```python
from build123d import *

# Parameters (mm, degrees)
SKETCH1_W           = 127
SKETCH1_H           = 87
BOSS_EXTRUDE1_DEPTH = 1.5
SKETCH3_W           = 131
SKETCH3_H           = 91
SKETCH3_W_2         = 127
SKETCH3_H_2         = 87
BOSS_EXTRUDE2_DEPTH = 20
CUT_EXTRUDE1_REACH  = 115.891
SKETCH4_W           = 25
SKETCH4_H           = 10
CUT_EXTRUDE2_REACH  = 142.112
SKETCH5_W           = 11
SKETCH5_H           = 10
CUT_EXTRUDE3_DEPTH  = 1.5


with BuildPart() as part:
    # Sketch1 → Boss-Extrude1 (new body)
    with BuildSketch(Plane(origin=(0, 0, 0), x_dir=(1, 0, 0), z_dir=(0, 1, 0))):
        Rectangle(SKETCH1_W, SKETCH1_H)
    extrude(amount=BOSS_EXTRUDE1_DEPTH)

    # Sketch3 → Boss-Extrude2 (add)
    with BuildSketch(Plane(origin=(0, 0, 0), x_dir=(1, 0, 0), z_dir=(0, 1, 0))):
        Rectangle(SKETCH3_W, SKETCH3_H)
        Rectangle(SKETCH3_W_2, SKETCH3_H_2, mode=Mode.SUBTRACT)
    extrude(amount=BOSS_EXTRUDE2_DEPTH)

    # Sketch4 → Cut-Extrude1 (cut, up to next)
    with BuildSketch(Plane.XY.offset(45.5), mode=Mode.PRIVATE) as cut_extrude1_sk1:
        with Locations((-45, 17)):
            Rectangle(SKETCH4_W, SKETCH4_H)
    cut_extrude1_tool1 = extrude(cut_extrude1_sk1.sketch, amount=-CUT_EXTRUDE1_REACH, mode=Mode.PRIVATE) & part.part
    add(cut_extrude1_tool1.solids().sort_by_distance((-45, 17, 45.5))[0], mode=Mode.SUBTRACT)

    # Sketch5 → Cut-Extrude2 (cut, up to next)
    with BuildSketch(Plane(origin=(65.5, 0, 0), x_dir=(0, 0, -1), z_dir=(1, 0, 0)), mode=Mode.PRIVATE) as cut_extrude2_sk1:
        with Locations((27.5, 11)):
            Rectangle(SKETCH5_W, SKETCH5_H)
    cut_extrude2_tool1 = extrude(cut_extrude2_sk1.sketch, amount=-CUT_EXTRUDE2_REACH, mode=Mode.PRIVATE) & part.part
    add(cut_extrude2_tool1.solids().sort_by_distance((65.5, 11, -27.5))[0], mode=Mode.SUBTRACT)

    # Sketch6 → Cut-Extrude3 (cut)
    with BuildSketch(Plane(origin=(0, 20, 0), x_dir=(1, 0, 0), z_dir=(0, 1, 0))):
        Polygon((-57.5, -44.5), (-64.5, -44.5), (-64.5, 44.5), (64.5, 44.5), (64.5, -44.5), (-32.5, -44.5), (-32.5, -45.5), (65.5, -45.5), (65.5, 45.5), (-65.5, 45.5), (-65.5, -45.5), (-57.5, -45.5), align=None)
    extrude(amount=-CUT_EXTRUDE3_DEPTH, mode=Mode.SUBTRACT)


solid = part.part
```
The listing builds one solid part. Answer for the finished solid, in the listing's coordinates (mm). A direction names the side the tool comes from. Coordinates: 2 decimals unless noted, no trailing zeros. Loops run counter-clockwise (first coordinate to the right, second up) from the corner with the lowest first, then second, coordinate; pieces in that order, holes last. Notation, with made-up numbers: (24, -35.75) - (30, -35.75) arc R4 cw to (30, -31.75) - close; hole circle Ø5 at (74.25, 76.25). An arc over 180 degrees is marked (long way). Use a Markdown table: item, result. Add a question column.
1) The part is cut by section C-C, the plane x = 49. Give the vertices of the cut face in (y, z).
2) The part is cut by section B-B, the plane z = -30.5. Give the vertices of the cut face in (x, y), and give its area (4 significant figures).
3) The part is cut by section D-D, the plane z = 4. Give the vertices of the cut face in (x, y).
4) The mould has two halves that part along Z. Classify faces 3 (the flat face through (-1, 9, 45.5)), 4 (the flat face through (-1, 0, -1)), 5 (the flat face through (63.5, 11, 1)): released by +Z, released by -Z, zero draft, split by the parting line, or undercut.
5) The part is cut by section A-A, the plane y = 13.75. Give the vertices of the cut face in (x, z), and give its area (3 significant figures).
6) Find the intervals of material crossed by line 1 (Z direction, x = 45, y = 17.25); line 2 (X direction, y = 9.25, z = 31); line 3 (Z direction, x = 35, y = 19), in increasing order.
7) Given pin 1 (2 mm diameter, centred on x = 28, z = -25, fed in from +Y); pin 2 (1.6 mm diameter, centred on y = 19.5, z = 8.5, fed in from +X); pin 3 (1.6 mm diameter, centred on x = -62, y = 19.5, fed in from +Z), each flat-ended and moving along its own axis, determine where each tip first touches the part or whether it passes through.
8) For faces 1 (the flat face through (-1, 11, 43.5)), 2 (the flat face through (-1, 9, -45.5)), determine the directions among +Z, -Z, +X, -X, +Y, -Y from which every point of the face is accessible in a straight line to the end or side of a thin tool.
Here are the results:
| question | item | result |
|---|---|---|
| 1 | outline | (0, -45.5) - (18.5, -45.5) - (18.5, -44.5) - (20, -44.5) - (20, -43.5) - (1.5, -43.5) - (1.5, 43.5) - (20, 43.5) - (20, 44.5) - (18.5, 44.5) - (18.5, 45.5) - (0, 45.5) - close |
| 2 | outline | (-65.5, 0) - (65.5, 0) - (65.5, 6) - (63.5, 6) - (63.5, 1.5) - (-63.5, 1.5) - (-63.5, 20) - (-64.5, 20) - (-64.5, 18.5) - (-65.5, 18.5) - close; (63.5, 16) - (65.5, 16) - (65.5, 18.5) - (64.5, 18.5) - (64.5, 20) - (63.5, 20) - close |
| 2 | area | 247.5 mm^2 |
| 3 | outline | (-65.5, 0) - (65.5, 0) - (65.5, 18.5) - (64.5, 18.5) - (64.5, 20) - (63.5, 20) - (63.5, 1.5) - (-63.5, 1.5) - (-63.5, 20) - (-64.5, 20) - (-64.5, 18.5) - (-65.5, 18.5) - close |
| 4 | face 3 | released by +Z |
| 4 | face 4 | zero draft |
| 4 | face 5 | undercut |
| 5 | outline | (-65.5, -45.5) - (65.5, -45.5) - (65.5, -33) - (63.5, -33) - (63.5, -43.5) - (-63.5, -43.5) - (-63.5, 43.5) - (-57.5, 43.5) - (-57.5, 45.5) - (-65.5, 45.5) - close; (-32.5, 43.5) - (63.5, 43.5) - (63.5, -22) - (65.5, -22) - (65.5, 45.5) - (-32.5, 45.5) - close |
| 5 | area | 800 mm^2 |
| 6 | line 1 | z = -45.5 to -43.5, 43.5 to 45.5 |
| 6 | line 2 | x = -65.5 to -63.5, 63.5 to 65.5 |
| 6 | line 3 | z = -44.5 to -43.5, 43.5 to 44.5 |
| 7 | pin 1 | stops at y = 1.5 |
| 7 | pin 2 | stops at x = 64.5 |
| 7 | pin 3 | stops at z = 44.5 |
| 8 | face 1 | +Y |
| 8 | face 2 | -Z, +X, -X, +Y, -Y |
